Verification items for the finished model (mm, model axes). Face numbers are marked on the shaded views. A direction names the side the tool comes from. Give positions to 0.01 mm unless a question says otherwise; leave off trailing zeros. Loops run counter-clockwise (first coordinate to the right, second up) from the corner with the lowest first, then second, coordinate; pieces in that order, holes last. Notation, with made-up numbers: (20.25, -32.75) - (31.25, -32.75) arc R17 cw to (31.25, -10.75) - close; hole circle Ø3 at (-20.75, 58). An arc over 180 degrees is marked (long way). One line per item, written item: value. Start each with the question number.
1. Mould release check, pull along X, two halves, no side actions. Record for the marked faces 3, 4 and 5: pulls with the +X half, pulls with the -X half, needs draft (parallel to the pull), parting line crosses it, or undercut.
2. Sectioned sample at B-B (x = -12.5). Record the cut outline in (y, z), plus the area to 3 significant figures.
3. Sectioned sample at C-C (y = -12). Record the cut outline in (x, z), plus the area to 3 significant figures.
4. Sectioned sample at A-A (z = 5.5). Record the cut outline in (x, y).
5. Gauge pin test, flat ends, axial feed: pin 1 (8 mm diameter, centred on x = 12.5, y = -12.5, fed in from -Z); pin 2 (17.5 mm diameter, centred on x = -3, y = 8.5, fed in from +Z). Record the tip position at first contact, or that the pin passes through.
6. Access from +Z, -Z, +X, -X, +Y, -Y to the whole of each face (thin tool, end or side, straight path). Record for the marked faces 1 and 2.
7. Sectioned sample at D-D (x = 5.5). Record the cut outline in (y, z).
8. Scan lines: L1, parallel to Y at x = -12.5, z = 3.4; L2, parallel to Y at x = -2, z = 6. Record each from-to range of solid material in increasing order. Write a range as [from, to].
from build123d import *

# Parameters (mm, degrees)
CROQUIS4_W              = 40
CROQUIS4_H              = 40
SALIENTE_EXTRUIR7_DEPTH = 5
CROQUIS5_W              = 40
CROQUIS5_H              = 40
CROQUIS5_W_2            = 35.003943974
CROQUIS5_H_2            = 35.003943974
SALIENTE_EXTRUIR8_DEPTH = 5
CROQUIS6_R              = 3.5
CORTAR_EXTRUIR1_DEPTH   = 13


with BuildPart() as part:
    # Croquis4 → Saliente-Extruir7 (new body)
    with BuildSketch(Plane.XY):
        Rectangle(CROQUIS4_W, CROQUIS4_H)
    extrude(amount=SALIENTE_EXTRUIR7_DEPTH)

    # Croquis5 → Saliente-Extruir8 (add)
    with BuildSketch(Plane.XY.offset(5)):
        Rectangle(CROQUIS5_W, CROQUIS5_H)
        Rectangle(CROQUIS5_W_2, CROQUIS5_H_2, mode=Mode.SUBTRACT)
    extrude(amount=SALIENTE_EXTRUIR8_DEPTH)

    # Croquis6 → Cortar-Extruir1 (cut)
    with BuildSketch(Plane.XY.offset(5)):
        with Locations((-12.5, 12.5)):
            Circle(CROQUIS6_R)
        with Locations((12.5, 12.5)):
            Circle(CROQUIS6_R)
        with Locations((-12.5, -12.5)):
            Circle(CROQUIS6_R)
        with Locations((12.5, -12.5)):
            Circle(CROQUIS6_R)
    extrude(amount=-CORTAR_EXTRUIR1_DEPTH, mode=Mode.SUBTRACT)


solid = part.part
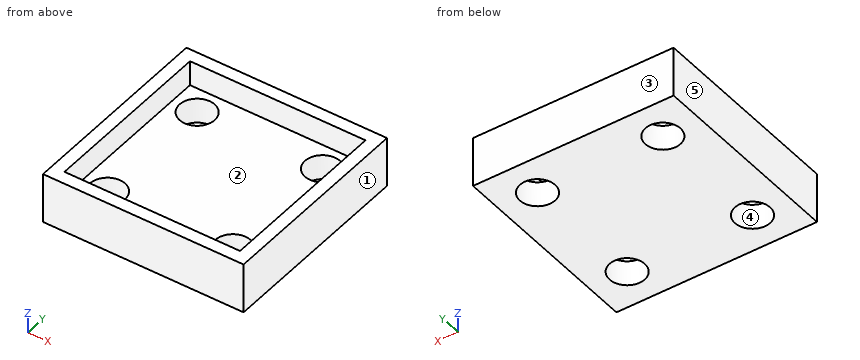
Results are:
1. face 3: needs draft
1. face 4: undercut
1. face 5: pulls with the -X half
2. outline: (-20, 0) - (-16, 0) - (-16, 5) - (-17.5, 5) - (-17.5, 10) - (-20, 10) - close; (-9, 0) - (9, 0) - (9, 5) - (-9, 5) - close; (16, 0) - (20, 0) - (20, 10) - (17.5, 10) - (17.5, 5) - (16, 5) - close
2. area: 155 mm^2
3. outline: (-20, 0) - (-15.96, 0) - (-15.96, 5) - (-17.5, 5) - (-17.5, 10) - (-20, 10) - close; (-9.04, 0) - (9.04, 0) - (9.04, 5) - (-9.04, 5) - close; (15.96, 0) - (20, 0) - (20, 10) - (17.5, 10) - (17.5, 5) - (15.96, 5) - close
3. area: 156 mm^2
4. outline: (-20, -20) - (20, -20) - (20, 20) - (-20, 20) - close; hole (-17.5, -17.5) - (17.5, -17.5) - (17.5, 17.5) - (-17.5, 17.5) - close
5. pin 1: stops at z = 0
5. pin 2: stops at z = 5
6. face 1: +Z, -Z, +X, +Y, -Y
6. face 2: +Z
7. outline: (-20, 0) - (20, 0) - (20, 10) - (17.5, 10) - (17.5, 5) - (-17.5, 5) - (-17.5, 10) - (-20, 10) - close
8. L1: y = [-20, -16], [-9, 9], [16, 20]
8. L2: y = [-20, -17.5], [17.5, 20]
